Autodesk Inventor part; units mm, degrees
ref_plane "YZ Plane" through (0, 0, 0) normal (1, 0, 0) x (0, 1, 0)
ref_plane "XZ Plane" through (0, 0, 0) normal (0, 1, 0) x (-1, 0, 0)
ref_plane "XY Plane" through (0, 0, 0) normal (0, 0, 1) x (1, 0, 0)
sketch "Эскиз1" plane through (0, 0, 0) normal (0, 1, 0) x (-1, 0, 0)
  line L0 (-127.5, 51.9915) -> (127.5, 51.9915)
  line L1 (127.5, 51.9915) -> (127.5, -51.9915)
  line L2 (127.5, -51.9915) -> (-127.5, -51.9915)
  line L3 (-127.5, -51.9915) -> (-127.5, 51.9915)
  line L4 (-48, 20) -> (48, 20)
  line L5 (48, 20) -> (48, -20)
  line L6 (48, -20) -> (-48, -20)
  line L7 (-48, -20) -> (-48, 20)
  line L8 (-48, 20) -> (48, -20) construction
  line L9 (48, 20) -> (-48, -20) construction
  line L10 (127.5, 19.4125) -> (110.25, 19.4125)
  line L11 (110.25, 19.4125) -> (110.25, -19.4125)
  line L12 (110.25, -19.4125) -> (127.5, -19.4125)
  line L13 (127.5, -19.4125) -> (127.5, 19.4125)
  line L14 (48, 0) -> (57.4345, 0)
  line L15 (0, 0) -> (0, -38.2708)
  line L16 (-127.5, 19.4125) -> (-110.25, 19.4125)
  line L17 (-110.25, 19.4125) -> (-110.25, -19.4125)
  line L18 (-110.25, -19.4125) -> (-127.5, -19.4125)
  line L19 (-127.5, -19.4125) -> (-127.5, 19.4125)
  dimension "d0" = 103.983
  dimension "d1" = 255
  dimension "d2" = 96
  dimension "d3" = 40
  dimension "d4" = 38.825
  dimension "d5" = 17.25
extrude "Выдавливание1" add sketch "Эскиз1" along normal blind 4 contours L0 L1 L10 L11 L12 L2 L3 L18 L17 L16
sketch "Эскиз2" plane through (0, 0, 0) normal (0, -1, 0) x (1, 0, 0)
  circle A0 centre (40, 36) radius 1.85
  circle A1 centre (40, -36) radius 1.85
  circle A2 centre (-40, -36) radius 1.85
  circle A3 centre (-40, 36) radius 1.85
  point P0 (0, 0)
extrude "Выдавливание2" cut sketch "Эскиз2" against normal blind 3
sketch "Эскиз3" plane through (0, 0, 0) normal (0, -1, 0) x (1, 0, 0)
  circle A0 centre (-106.875, 18.5) radius 1.5
  circle A1 centre (-69.875, 18.5) radius 1.5
  circle A2 centre (-106.875, -18.5) radius 1.5
  circle A3 centre (-69.875, -18.5) radius 1.5
  circle A4 centre (69.875, -18.5) radius 1.5
  circle A5 centre (69.875, 18.5) radius 1.5
  circle A6 centre (106.875, 18.5) radius 1.5
  circle A7 centre (106.875, -18.5) radius 1.5
  point P0 (0, 0)
extrude "Выдавливание3" cut sketch "Эскиз3" against normal blind 4
chamfer "Фаска1" distance 2 angle 45 8 edges at (-108.375, 4, 18.5) (-71.375, 4, 18.5) (-71.375, 4, -18.5) (-108.375, 4, -18.5) (68.375, 4, -18.5) (68.375, 4, 18.5) (105.375, 4, 18.5) (105.375, 4, -18.5)
properties part number "KB33-046-004-019 - Площадка под драйверы"
Could you check a few things on this model? Use its own coordinates, in mm. Round coordinates to 2 decimals unless told otherwise and drop trailing zeros. Write each loop counter-clockwise with the first axis right and the second up, starting at its lowest first coordinate (ties: lowest second). Pieces come first, ordered by that corner, then holes. Notation, with made-up numbers: (-13, 85) - (29, 85) arc R11 cw to (29, 103) - close; hole circle Ø10 at (63.25, -15). An arc over 180 degrees is marked (long way). Use a Markdown table: item, result.
Q1. I want a section at B-B (x = 1.5). List the corners of the cut face in (y, z) for me, plus the area to 3 significant figures.
Output values:
| item | result |
|---|---|
| outline | (0, -51.99) - (4, -51.99) - (4, -20) - (0, -20) - close; (0, 20) - (4, 20) - (4, 51.99) - (0, 51.99) - close |
| area | 256 mm2 |
Q2. For pin 1 (1.8 mm diameter, centred on x = 69.875, z = 18.5, fed in from -Y); pin 2 (3.5 mm diameter, centred on x = -69.875, z = -18.5, fed in from +Y); pin 3 (1.1 mm diameter, centred on x = -39.5, z = -36.5, fed in from -Y), each with a flat end and sliding along its axis, tell me the tip position at first contact or that it passes through.
Output values:
| item | result |
|---|---|
| pin 1 | through |
| pin 2 | y = 2.25 |
| pin 3 | y = 3 |
Q3. Thinking about a two-plate mould opening in Z: for faces 1 (the conical face through (108.43, 2.13, -18.99)), 2 (the conical face through (-105.32, 2.13, 18.01)), 3 (the flat face through (2, 0, -22)), which applies, released by +Z, released by -Z, zero draft, split by the parting line, or undercut?
Output values:
| item | result |
|---|---|
| face 1 | undercut |
| face 2 | undercut |
| face 3 | zero draft |
Q4. Please list where these lines run through material, in increasing order: L1, parallel to Z at x = 40, y = 1.95; L2, parallel to Z at x = -28, y = 2.9; L3, parallel to Z at x = 116.5, y = 2.3.
Output values:
| item | result |
|---|---|
| L1 | -51.99 to -37.85, -34.15 to -20, 20 to 34.15, 37.85 to 51.99 |
| L2 | -51.99 to -20, 20 to 51.99 |
| L3 | -51.99 to -19.41, 19.41 to 51.99 |
Q5. I want a section at A-A (z = -9.5). List the corners of the cut face in (x, y) for me.
Output values:
| item | result |
|---|---|
| outline | (-110.25, 0) - (-48, 0) - (-48, 4) - (-110.25, 4) - close; (48, 0) - (110.25, 0) - (110.25, 4) - (48, 4) - close |
